from build123d import *

# Parameters (mm, degrees)
F0_W     = 1000
F0_H     = 700
F1_DEPTH = 10
F2_W     = 900
F2_H     = 600
F2_W_2   = 800
F2_H_2   = 500
F3_DEPTH = 5
F4_W     = 900
F4_H     = 600
F4_W_2   = 890
F4_H_2   = 590
F5_DEPTH = 50
F7_DEPTH = 1000


with BuildPart() as f1:
    # F0 (on Top) → F1 (new body)
    with BuildSketch(Plane.XY):
        with Locations((440.967437, 309.230214)):
            Rectangle(F0_W, F0_H)
    extrude(amount=-F1_DEPTH)

    # F2 (on face) → F3 (join)
    with BuildSketch(Plane(origin=(0, 0, -10), x_dir=(1, 0, 0), z_dir=(0, 0, -1))):
        with Locations((440.967437, -309.230214)):
            Rectangle(F2_W, F2_H)
        with Locations((440.967437, -309.230214)):
            Rectangle(F2_W_2, F2_H_2, mode=Mode.SUBTRACT)
    extrude(amount=F3_DEPTH)

    # F4 (on face) → F5 (join)
    with BuildSketch(Plane(origin=(0, 0, -15), x_dir=(1, 0, 0), z_dir=(0, 0, -1))):
        with Locations((440.967437, -309.230214)):
            Rectangle(F4_W, F4_H)
        with Locations((440.967437, -309.230214)):
            Rectangle(F4_W_2, F4_H_2, mode=Mode.SUBTRACT)
    extrude(amount=F5_DEPTH)

    # F6 (on face) → F7 (join)
    with BuildSketch(Plane(origin=(0, 0, -10), x_dir=(1, 0, 0), z_dir=(0, 0, -1))):
        Polygon((-9.032563, -59.230214), (-9.032563, -9.230214), (40.967437, -9.230214), (40.967437, -4.230214), (-14.032563, -4.230214), (-14.032563, -59.230214), align=None)
        Polygon((40.967437, -609.230214), (-9.032563, -609.230214), (-9.032563, -559.230214), (-14.032563, -559.230214), (-14.032563, -614.230214), (40.967437, -614.230214), align=None)
        Polygon((840.967437, -14.230214), (890.967437, -14.230214), (890.967437, -64.230214), (895.967437, -64.230214), (895.967437, -9.230214), (840.967437, -9.230214), align=None)
        Polygon((890.967437, -559.230214), (890.967437, -609.230214), (840.967437, -609.230214), (840.967437, -614.230214), (895.967437, -614.230214), (895.967437, -559.230214), align=None)
    extrude(amount=F7_DEPTH)


solid = f1.part
Design review of the part built by this model. Coordinates are the model's own, in mm. A direction names the side the tool comes from. Give positions to 0.01 mm unless a question says otherwise; leave off trailing zeros. Order: outer loops, then holes, each group sorted by start corner. A loop starts at its lowest first (then second) coordinate and runs counter-clockwise, first axis right, second up.
1. Add section C-C, the plane x = 502. State the section outline as (y, z) points, then the cut area to 3 significant figures.
Solution:
outline: (-40.77, -10) - (9.23, -10) - (9.23, -65) - (14.23, -65) - (14.23, -15) - (59.23, -15) - (59.23, -10) - (559.23, -10) - (559.23, -15) - (604.23, -15) - (604.23, -65) - (609.23, -65) - (609.23, -10) - (659.23, -10) - (659.23, 0) - (-40.77, 0) - close
area: 8,000 mm2
2. Mouldability with a two-part tool opening along Y and no side actions: class faces 1 (the flat face through (13, 614.23, -503)), 2 (the flat face through (879, 14, -1010)), 3 (the flat face through (890.967, 39, -531)) as +Y half, -Y half, draft (parallel to the pull), parting line (faces both ways), or undercut.
Solution:
face 1: +Y half
face 2: draft
face 3: undercut
3. Add section B-B, the plane z = -232. State the section outline as (x, y) points.
Solution:
outline: (-14.03, 4.23) - (40.97, 4.23) - (40.97, 9.23) - (-9.03, 9.23) - (-9.03, 59.23) - (-14.03, 59.23) - close; (-14.03, 559.23) - (-9.03, 559.23) - (-9.03, 609.23) - (40.97, 609.23) - (40.97, 614.23) - (-14.03, 614.23) - close; (840.97, 9.23) - (895.97, 9.23) - (895.97, 64.23) - (890.97, 64.23) - (890.97, 14.23) - (840.97, 14.23) - close; (840.97, 609.23) - (890.97, 609.23) - (890.97, 559.23) - (895.97, 559.23) - (895.97, 614.23) - (840.97, 614.23) - close
4. To check wall thickness, follow L1, parallel to X at y = 32, z = -237.5; L2, parallel to Y at x = 39.5, z = -764; L3, parallel to Y at x = 871, z = -167. State the ranges of each line that lie inside material, in increasing order.
Solution:
L1: x = -14.03 to -9.03, 890.97 to 895.97
L2: y = 4.23 to 9.23, 609.23 to 614.23
L3: y = 9.23 to 14.23, 609.23 to 614.23
5. Add section A-A, the plane y = 575. State the section outline as (x, z) points.
Solution:
outline: (-59.03, -10) - (-14.03, -10) - (-14.03, -1010) - (-9.03, -1010) - (-9.03, -65) - (-4.03, -65) - (-4.03, -15) - (885.97, -15) - (885.97, -65) - (890.97, -65) - (890.97, -1010) - (895.97, -1010) - (895.97, -10) - (940.97, -10) - (940.97, 0) - (-59.03, 0) - close
6. Tool access review of faces 4 (the flat face through (16, 9.23, -531)), 5 (the flat face through (868, 614.23, -503)), 6 (the flat face through (890.967, 315, -37)), 7 (the flat face through (-14.033, 586, -503)): name each direction out of +Z, -Z, +X, -X, +Y, -Y from which nothing blocks a thin tool from reaching the whole face with its end or side.
Solution:
face 4: -Z
face 5: -Z, +X, -X, +Y
face 6: -Z, +X
face 7: -Z, -X, +Y, -Y
7. For pin 1 Ø5 at (x, y) = (293, 199) entering from -Z; pin 2 Ø2.5 at (x, z) = (291.5, -13.5) entering from -Y; pin 3 Ø16.5 at (y, z) = (583.5, -540.5) entering from -X, all flat-tipped, find the tip position at first contact; note any pin that passes through.
Solution:
pin 1: stops at z = -10
pin 2: stops at y = 9.23
pin 3: stops at x = -14.03
